Design review of the part built by this model. Coordinates are the model's own, in mm. A direction names the side the tool comes from. Round coordinates to 2 decimals unless told otherwise and drop trailing zeros. Order: outer loops, then holes, each group sorted by start corner. A loop starts at its lowest first (then second) coordinate and runs counter-clockwise, first axis right, second up. Notation, with made-up numbers: M 26.25,79.5 L 60.25,79.5 A28 cw 60.25,109.5 Z; hole C 84.5,64 d11. An arc over 180 degrees is marked long. Write item = value, one per line. Start each with the question number.
```python
from build123d import *

# Parameters (mm, degrees)
F0_W      = 290.640860796
F0_H      = 330.3228616714
F1_DEPTH  = 25.4
F2_W      = 254.641264677
F2_H      = 304.1897118092
F3_DEPTH  = 25.4
F4_W      = 195.6849247217
F4_H      = 247.7421462536
F5_DEPTH  = 101.6
F6_W      = 180.6322485209
F6_H      = 228.9262861013
F7_DEPTH  = 25.4
F7_TAPER  = -3
F8_W      = 137.9829794168
F8_H      = 183.7682276964
F9_DEPTH  = 25.4
F9_TAPER  = -10
F10_W     = 82.7897712588
F10_H     = 121.0486963391
F11_DEPTH = 25.4
F11_TAPER = -3
F12_DEPTH = 132.08
F13_DEPTH = 99.06
F14_DEPTH = 83.82
F15_DEPTH = 254


with BuildPart() as f1:
    # F0 (on Top) → F1 (new body)
    with BuildSketch(Plane.XY):
        Rectangle(F0_W, F0_H)
    extrude(amount=F1_DEPTH)

    # F2 (on face) → F3 (join)
    with BuildSketch(Plane.XY.offset(25.4)):
        Rectangle(F2_W, F2_H)
    extrude(amount=F3_DEPTH)

    # F4 (on face) → F5 (join)
    with BuildSketch(Plane.XY.offset(50.8)):
        Rectangle(F4_W, F4_H)
    extrude(amount=F5_DEPTH)

    # F6 (on face) → F7 (cut)
    with BuildSketch(Plane.XY.offset(152.4)):
        Rectangle(F6_W, F6_H)
    extrude(amount=-F7_DEPTH, taper=F7_TAPER, mode=Mode.SUBTRACT)

    # F8 (on face) → F9 (cut)
    with BuildSketch(Plane.XY.offset(127)):
        Rectangle(F8_W, F8_H)
    extrude(amount=-F9_DEPTH, taper=F9_TAPER, mode=Mode.SUBTRACT)

    # F10 (on face) → F11 (cut)
    with BuildSketch(Plane.XY.offset(101.6)):
        Rectangle(F10_W, F10_H)
    extrude(amount=-F11_DEPTH, taper=F11_TAPER, mode=Mode.SUBTRACT)

    # F12 (add): a face of the model
    f12_faces = [f1.faces().sort_by_distance(p)[0] for p in [
        (0, -123.8710731268, 101.6),
    ]]
    extrude(f12_faces, amount=F12_DEPTH)

    # F13 (add): a face of the model
    f13_faces = [f1.faces().sort_by_distance(p)[0] for p in [
        (0, -148.8583176808, 152.4),
    ]]
    extrude(f13_faces, amount=F13_DEPTH)

    # F14 (add): a face of the model
    f14_faces = [f1.faces().sort_by_distance(p)[0] for p in [
        (0, -148.8583176808, 251.46),
    ]]
    extrude(f14_faces, amount=F14_DEPTH)

    # F15 (add): a face of the model
    f15_faces = [f1.faces().sort_by_distance(p)[0] for p in [
        (0, -255.9510731268, 193.04),
    ]]
    extrude(f15_faces, amount=F15_DEPTH)


solid = f1.part
```
(1) Insertion check: pin 1 (3 mm diameter, centred on x = -24, z = 49, fed in from -Y); pin 2 (12 mm diameter, centred on x = 102, z = 251.5, fed in from +Y); pin 3 (2 mm diameter, centred on y = -434.5, z = 143.5, fed in from -X); pin 4 (20.5 mm diameter, centred on x = 63.5, z = 35, fed in from +Y). Each pin has a flat end and moves straight along its axis. Give the tip position at first contact, or say it passes through.
(2) Consider section C-C, the plane y = -241.5. Write out the cut boundary in (x, z), then the cut area to 3 significant figures.
(3) For line 1 along X through (y, z) = (37, 221.5); line 2 along Y through (x, z) = (-82, 238.5); line 3 along Z through (x, y) = (-14.5, -159.5), list the stretches that pass through material, from the lowest coordinate up. Write a range as [from, to].
(4) Draft analysis for pull direction Y (two halves, no side actions). For faces 1 (the face through (-70, -1, 127)), 2 (the face through (-1, 123.871, 191)), 3 (the face through (97.842, -189, 191)), state which applies: pulls with the +Y half, pulls with the -Y half, needs draft (parallel to the pull), parting line crosses it, or undercut.
(5) Consider section A-A, the plane z = 300. Write out the cut boundary in (x, y), then the cut area to 3 significant figures.
(6) Consider section B-B, the plane x = 115.5. Write out the cut boundary in (y, z).
(7) For faces 4 (the face through (-2, -152.095, 38)), 5 (the face through (-1, -114.463, 243)), 6 (the face through (-127.321, -2, 38)), list the 3-axis set-ups (+Z, -Z, +X, -X, +Y, -Y) from which the entire face can be reached by the end or side of a thin tool; tool diameter is ignored.
Completed:
q1.pin_1 = -152.09
q1.pin_2 = 123.87
q1.pin_3 = -97.84
q1.pin_4 = 165.16
q2.outline = M -97.84,50.8 L 97.84,50.8 L 97.84,335.28 L -97.84,335.28 Z
q2.area = 55,700 mm2
q3.line_1 = [-97.84, -90.32], [90.32, 97.84]
q3.line_2 = [-509.95, -114.46], [114.46, 123.87]
q3.line_3 = [0, 25.4], [50.8, 335.28]
q4.face_1 = undercut
q4.face_2 = pulls with the +Y half
q4.face_3 = needs draft
q5.outline = M -97.84,-509.95 L 97.84,-509.95 L 97.84,123.87 L -97.84,123.87 Z; hole M -90.32,-114.46 L 90.32,-114.46 L 90.32,114.46 L -90.32,114.46 Z
q5.area = 82,700 mm2
q6.outline = M -165.16,0 L 165.16,0 L 165.16,25.4 L 152.09,25.4 L 152.09,50.8 L -152.09,50.8 L -152.09,25.4 L -165.16,25.4 Z
q7.face_4 = +X, -X, -Y
q7.face_5 = +Z
q7.face_6 = +Z, -X, +Y, -Y
